Here's the drawing with two shaded views (mm, measured from the low corner). I have some questions. Give positions to 0.01 mm unless a question says otherwise; leave off trailing zeros. Write each loop counter-clockwise with the first axis right and the second up, starting at its lowest first coordinate (ties: lowest second). Pieces come first, ordered by that corner, then holes. Notation, with made-up numbers: M -4.75,-11.5 L 17.25,-11.5 A24 cw 17.25,22.5 Z; hole C 14.25,75.5 d6. An arc over 180 degrees is marked long. Use one line per item in the form item = value. Start each with the question number.
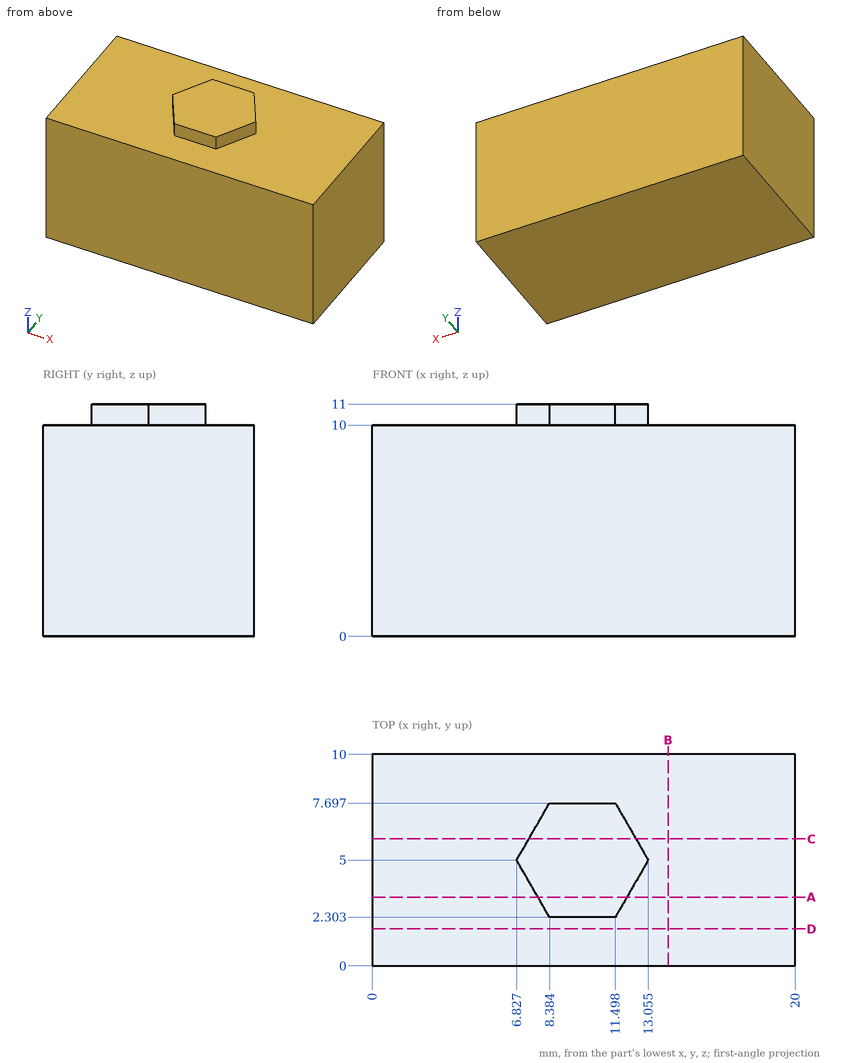
1) Suppose I cut it at B-B, the plane x = 14. List the corners of the cut face in (y, z) for me, and give its area (3 significant figures).
2) Please list where this line runs through material, in increasing order: line 1 (Z direction, x = 18.75, y = 6.25).
3) Suppose I cut it at A-A, the plane y = 3.25. List the corners of the cut face in (x, z) for me (1 decimal).
4) Suppose I cut it at D-D, the plane y = 1.75. List the corners of the cut face in (x, z) for me, and give its area (3 significant figures).
5) Suppose I cut it at C-C, the plane y = 6. List the corners of the cut face in (x, z) for me (1 decimal), and give its area (3 significant figures).
6) Will these pins go through, and if not, where does the flat tip stop? P1, Ø1.5, axis at x = 3.5, y = 1, coming from the +Z side; P2, Ø1, axis at x = 17, y = 2, coming from the -Z side; P3, Ø0.5, axis at x = 10.5, z = 10.5, coming from the +Y side.
Checks:
q1.outline = M 0,0 L 10,0 L 10,10 L 0,10 Z
q1.area = 100 mm^2
q2.line_1 = 0 to 10
q3.outline = M 0,0 L 20,0 L 20,10 L 12,10 L 12,11 L 7.8,11 L 7.8,10 L 0,10 Z
q4.outline = M 0,0 L 20,0 L 20,10 L 0,10 Z
q4.area = 200 mm^2
q5.outline = M 0,0 L 20,0 L 20,10 L 12.5,10 L 12.5,11 L 7.4,11 L 7.4,10 L 0,10 Z
q5.area = 205 mm^2
q6.P1 = 10
q6.P2 = 0
q6.P3 = 7.7
